Geometry check sheet. Reference: the model listing, model coordinates, mm. Face numbers are marked on the shaded views. A direction names the side the tool comes from. Round coordinates to 2 decimals unless told otherwise and drop trailing zeros. Write each loop counter-clockwise with the first axis right and the second up, starting at its lowest first coordinate (ties: lowest second). Pieces come first, ordered by that corner, then holes.
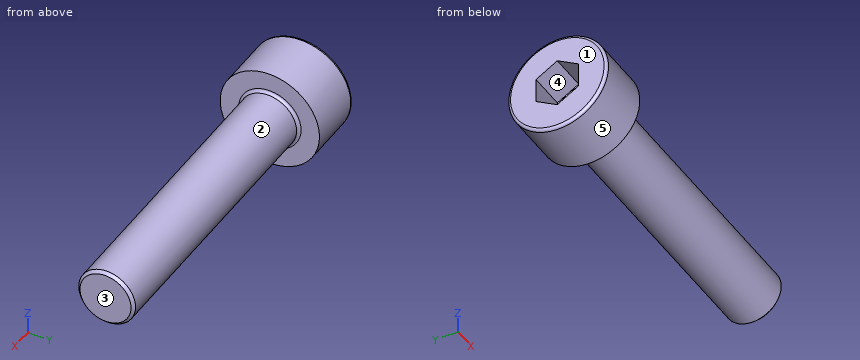
from build123d import *

# Parameters (mm, degrees)
HOLE_WIZARD_3_0_3_1_D     = 3
HOLE_WIZARD_3_0_3_1_DEPTH = 2.6
HOLE_WIZARD_3_0_3_1_TIP   = 0.901290929
CUT_EXTRUDE_1_DEPTH       = 2.6
FILLET_1_R                = 0.2
CHAMFER_1_SIZE            = 0.2


with BuildPart() as part:
    # 草图1 → 旋转1 (revolve)
    with BuildSketch(Plane.XY):
        Polygon((0, 0), (0, 3.5), (4, 3.5), (4, 2), (24, 2), (24, 0), align=None)
    revolve(axis=Axis((0, 0, 0), (1, 0, 0)))

    # Ø3.0 (3) 直径孔1
    with Locations(Plane.ZY):
        with Locations((0, 0)):
            Hole(HOLE_WIZARD_3_0_3_1_D / 2, depth=HOLE_WIZARD_3_0_3_1_DEPTH)
            with Locations((0, 0, -(HOLE_WIZARD_3_0_3_1_DEPTH + HOLE_WIZARD_3_0_3_1_TIP / 2))):  # 118° drill point
                Cone(0, HOLE_WIZARD_3_0_3_1_D / 2, HOLE_WIZARD_3_0_3_1_TIP, mode=Mode.SUBTRACT)

    # 草图2 → 切除-拉伸1 (cut)
    with BuildSketch(Plane.ZY):
        Polygon((0.866025404, 1.5), (-0.866025404, 1.5), (-1.732050808, 0), (-0.866025404, -1.5), (0.866025404, -1.5), (1.732050808, 0), align=None)
    extrude(amount=-CUT_EXTRUDE_1_DEPTH, mode=Mode.SUBTRACT)

    # 圆角1
    fillet_1_edges = [part.edges().sort_by_distance(p)[0] for p in [
        (4, -2, 0),
        (0, -3.5, 0),
    ]]
    fillet(fillet_1_edges, radius=FILLET_1_R)

    # 倒角1
    chamfer_1_edges = [part.edges().sort_by_distance(p)[0] for p in [
        (24, -2, 0),
    ]]
    chamfer(chamfer_1_edges, length=CHAMFER_1_SIZE)


solid = part.part
1. Section check A-A (x = 14). Record the cut outline in (y, z).
2. Access from +Z, -Z, +X, -X, +Y, -Y to the whole of each face (thin tool, end or side, straight path). Record for the marked faces 1 and 2.
3. Depth check by flat-ended pin: pin 1 Ø4 at (x, z) = (20, -1) entering from +Y; pin 2 Ø2 at (x, z) = (8.5, 1.5) entering from +Y. Enter the tip coordinate at first touch or a pass-through.
4. Scan lines: line 1 along X through (y, z) = (1, 2); line 2 along Z through (x, y) = (23, -0.5); line 3 along X through (y, z) = (0.25, -0.25). Record each from-to range of solid material in increasing order.
5. Release check for a two-part mould opening along Y. For the marked faces 3, 4 and 5 record: +Y half, -Y half, draft (parallel to the pull), parting line (faces both ways), or undercut.
Results below:
1. outline: circle Ø4 at (0, 0)
2. face 1: +Z, -Z, -X, +Y, -Y
2. face 2: +X
3. pin 1: stops at y = 2
3. pin 2: stops at y = 1.94
4. line 1: x = 0 to 4
4. line 2: z = -1.94 to 1.94
4. line 3: x = 3.29 to 24
5. face 3: draft
5. face 4: undercut
5. face 5: parting line
